Can you work these out from the model? Positions are in its coordinate system, mm. A direction names the side the tool comes from. Give positions to 0.01 mm unless a question says otherwise; leave off trailing zeros. Order: outer loops, then holes, each group sorted by start corner. A loop starts at its lowest first (then second) coordinate and runs counter-clockwise, first axis right, second up. Notation, with made-up numbers: M -12,9 L 32,9 A16 cw 32,36 Z; hole C 11,-28 d1. An arc over 180 degrees is marked long. Use one line per item in the form item = value. Start each with the question number.
1. I want a section at B-B, the plane y = 149. List the corners of the cut face in (x, z) for me (3 decimals).
2. We'd pull the mould along Y, two halves only. Please class faces 6 (the face through (134, 184, 69.85)), 7 (the face through (134, 5.588, 60)), 8 (the face through (134, 12.668, -67)): +Y half, -Y half, draft (parallel to the pull), parting line (faces both ways), or undercut.
3. I want a section at C-C, the plane x = 134.2. Count the separate pieces of the cut face and the enclosed holes in it, and give its area (3 significant figures).
4. I need wall thicknesses on L1, parallel to Y at x = 134, z = 50.8; L2, parallel to Y at x = 134.1, z = 8; L3, parallel to Y at x = 135.45, z = -28.5. Which ranges of each line are inside material? Lowest first, please.
5. I want a section at A-A, the plane y = 34.5. List the corners of the cut face in (x, z) for me (3 decimals), and give its area (3 significant figures).
6. Will these pins go through, and if not, where does the flat tip stop? P1, Ø3, axis at x = 134.5, y = 273.5, coming from the +Z side; P2, Ø1.7, axis at x = 133.5, y = 173, coming from the -Z side; P3, Ø3, axis at x = 133, z = -67, coming from the +Y side.
7. For faces 1 (the face through (134, 24, -30.988)), 2 (the face through (134, 196, 63.5)), 3 (the face through (134, 3, -57.15)), 4 (the face through (134, 108, -69.85)), 5 (the face through (134, 126.682, -67)), which set-ups out of +Z, -Z, +X, -X, +Y, -Y let a thin tool reach every point of the face, with its end or its side?
```python
from build123d import *

# Parameters (mm, degrees)
SKETCH1_W              = 273.05
SKETCH1_H              = 139.7
BOSS_EXTRUDE1_DEPTH    = 5.588
SKETCH2_W              = 273.05
SKETCH2_H              = 139.7
SKETCH2_W_2            = 261.874
SKETCH2_H_2            = 128.524
BOSS_EXTRUDE2_DEPTH    = 298.45
SKETCH3_W              = 6.35
SKETCH3_H              = 16.933333333
SKETCH3_H_2            = 16.933333334
DOOR_SLOT_DEPTH        = 12.7
DOOR_GUIDE_HOLES_REACH = 361.255
SKETCH4_W              = 6.35
SKETCH4_H              = 15.875
LEVER_HOLES_W          = 9.652
LEVER_HOLES_H          = 6.35
LEVER_HOLES_W_2        = 6.35
CUT_EXTRUDE1_DEPTH     = 362.378293578
CUT_EXTRUDE3_REACH     = 416.577
SKETCH8_R              = 3.175
SKETCH16_W             = 327.238778096
SKETCH16_H             = 314.471565403
CUT_EXTRUDE10_DEPTH    = 362.378293578
LEFT_RIGHT_W           = 6.35
LEFT_RIGHT_H           = 5.588
LEFT_RIGHT_W_2         = 12.7
LEFT_RIGHT_H_2         = 12.66825
CUT_EXTRUDE11_DEPTH    = 415.577411883
SKETCH17_R             = 1.5
SKETCH17_W             = 23
SKETCH17_H             = 17.61800007
CUT_EXTRUDE12_DEPTH    = 313.00857951
SKETCH18_W             = 5.588
SKETCH18_H             = 12.192
CUT_EXTRUDE13_DEPTH    = 313.00857951


with BuildPart() as part:
    # Sketch1 → Boss-Extrude1 (new body)
    with BuildSketch(Plane(origin=(0, 0, 0), x_dir=(1, 0, 0), z_dir=(0, 1, 0))):
        Rectangle(SKETCH1_W, SKETCH1_H)
    extrude(amount=BOSS_EXTRUDE1_DEPTH)

    # Sketch2 → Boss-Extrude2 (add)
    with BuildSketch(Plane(origin=(0, 5.588, 0), x_dir=(1, 0, 0), z_dir=(0, 1, 0))):
        Rectangle(SKETCH2_W, SKETCH2_H)
        Rectangle(SKETCH2_W_2, SKETCH2_H_2, mode=Mode.SUBTRACT)
    extrude(amount=BOSS_EXTRUDE2_DEPTH)

    # Sketch3 → Door Slot (cut)
    with BuildSketch(Plane.XY.offset(69.85)):
        with BuildLine():
            Line((-29.337, 282.448), (-29.337, 5.588))
            Line((-29.337, 5.588), (-22.733, 5.588))
            Line((-22.733, 5.588), (-22.733, 291.592))
            Line((-22.733, 291.592), (-42.291, 291.592))
            Line((-42.291, 291.592), (-42.291, 284.988))
            Line((-42.291, 284.988), (-31.877, 284.988))
            ThreePointArc((-31.877, 284.988), (-30.080948776, 284.244051224), (-29.337, 282.448))
        make_face()
        with Locations((-13.208, 80.433333334)):
            Rectangle(SKETCH3_W, SKETCH3_H)
        with Locations((-13.208, 50.8)):
            Rectangle(SKETCH3_W, SKETCH3_H_2)
        with Locations((-13.208, 21.166666667)):
            Rectangle(SKETCH3_W, SKETCH3_H)
    extrude(amount=-DOOR_SLOT_DEPTH, mode=Mode.SUBTRACT)

    # Sketch4 → Door Guide Holes (cut, up to next)
    with BuildSketch(Plane.XY.offset(-64.262), mode=Mode.PRIVATE) as door_guide_holes_sk1:
        with Locations((-45.466, 283.4005)):
            Rectangle(SKETCH4_W, SKETCH4_H)
    door_guide_holes_tool1 = extrude(door_guide_holes_sk1.sketch, amount=-DOOR_GUIDE_HOLES_REACH, mode=Mode.PRIVATE) & part.part
    # Sketch4 → Door Guide Holes (cut, up to next)
    with BuildSketch(Plane.XY.offset(-64.262), mode=Mode.PRIVATE) as door_guide_holes_sk2:
        with Locations((-45.466, 254.8255)):
            Rectangle(SKETCH4_W, SKETCH4_H)
    door_guide_holes_tool2 = extrude(door_guide_holes_sk2.sketch, amount=-DOOR_GUIDE_HOLES_REACH, mode=Mode.PRIVATE) & part.part
    # Sketch4 → Door Guide Holes (cut, up to next)
    with BuildSketch(Plane.XY.offset(-64.262), mode=Mode.PRIVATE) as door_guide_holes_sk3:
        with Locations((-45.466, 226.2505)):
            Rectangle(SKETCH4_W, SKETCH4_H)
    door_guide_holes_tool3 = extrude(door_guide_holes_sk3.sketch, amount=-DOOR_GUIDE_HOLES_REACH, mode=Mode.PRIVATE) & part.part
    # Sketch4 → Door Guide Holes (cut, up to next)
    with BuildSketch(Plane.XY.offset(-64.262), mode=Mode.PRIVATE) as door_guide_holes_sk4:
        with Locations((-45.466, 197.6755)):
            Rectangle(SKETCH4_W, SKETCH4_H)
    door_guide_holes_tool4 = extrude(door_guide_holes_sk4.sketch, amount=-DOOR_GUIDE_HOLES_REACH, mode=Mode.PRIVATE) & part.part
    # Sketch4 → Door Guide Holes (cut, up to next)
    with BuildSketch(Plane.XY.offset(-64.262), mode=Mode.PRIVATE) as door_guide_holes_sk5:
        with Locations((-45.466, 169.1005)):
            Rectangle(SKETCH4_W, SKETCH4_H)
    door_guide_holes_tool5 = extrude(door_guide_holes_sk5.sketch, amount=-DOOR_GUIDE_HOLES_REACH, mode=Mode.PRIVATE) & part.part
    # Sketch4 → Door Guide Holes (cut, up to next)
    with BuildSketch(Plane.XY.offset(-64.262), mode=Mode.PRIVATE) as door_guide_holes_sk6:
        with Locations((-45.466, 140.5255)):
            Rectangle(SKETCH4_W, SKETCH4_H)
    door_guide_holes_tool6 = extrude(door_guide_holes_sk6.sketch, amount=-DOOR_GUIDE_HOLES_REACH, mode=Mode.PRIVATE) & part.part
    # Sketch4 → Door Guide Holes (cut, up to next)
    with BuildSketch(Plane.XY.offset(-64.262), mode=Mode.PRIVATE) as door_guide_holes_sk7:
        with Locations((-45.466, 111.9505)):
            Rectangle(SKETCH4_W, SKETCH4_H)
    door_guide_holes_tool7 = extrude(door_guide_holes_sk7.sketch, amount=-DOOR_GUIDE_HOLES_REACH, mode=Mode.PRIVATE) & part.part
    # Sketch4 → Door Guide Holes (cut, up to next)
    with BuildSketch(Plane.XY.offset(-64.262), mode=Mode.PRIVATE) as door_guide_holes_sk8:
        with Locations((-45.466, 83.3755)):
            Rectangle(SKETCH4_W, SKETCH4_H)
    door_guide_holes_tool8 = extrude(door_guide_holes_sk8.sketch, amount=-DOOR_GUIDE_HOLES_REACH, mode=Mode.PRIVATE) & part.part
    # Sketch4 → Door Guide Holes (cut, up to next)
    with BuildSketch(Plane.XY.offset(-64.262), mode=Mode.PRIVATE) as door_guide_holes_sk9:
        with Locations((-45.466, 54.8005)):
            Rectangle(SKETCH4_W, SKETCH4_H)
    door_guide_holes_tool9 = extrude(door_guide_holes_sk9.sketch, amount=-DOOR_GUIDE_HOLES_REACH, mode=Mode.PRIVATE) & part.part
    # Sketch4 → Door Guide Holes (cut, up to next)
    with BuildSketch(Plane.XY.offset(-64.262), mode=Mode.PRIVATE) as door_guide_holes_sk10:
        with Locations((-45.466, 26.2255)):
            Rectangle(SKETCH4_W, SKETCH4_H)
    door_guide_holes_tool10 = extrude(door_guide_holes_sk10.sketch, amount=-DOOR_GUIDE_HOLES_REACH, mode=Mode.PRIVATE) & part.part
    door_guide_holes_1 = door_guide_holes_tool1.solids().sort_by_distance((-45.466, 283.4005, -64.262))[0]
    add(door_guide_holes_1, mode=Mode.SUBTRACT)
    door_guide_holes_2 = door_guide_holes_tool2.solids().sort_by_distance((-45.466, 254.8255, -64.262))[0]
    add(door_guide_holes_2, mode=Mode.SUBTRACT)
    door_guide_holes_3 = door_guide_holes_tool3.solids().sort_by_distance((-45.466, 226.2505, -64.262))[0]
    add(door_guide_holes_3, mode=Mode.SUBTRACT)
    door_guide_holes_4 = door_guide_holes_tool4.solids().sort_by_distance((-45.466, 197.6755, -64.262))[0]
    add(door_guide_holes_4, mode=Mode.SUBTRACT)
    door_guide_holes_5 = door_guide_holes_tool5.solids().sort_by_distance((-45.466, 169.1005, -64.262))[0]
    add(door_guide_holes_5, mode=Mode.SUBTRACT)
    door_guide_holes_6 = door_guide_holes_tool6.solids().sort_by_distance((-45.466, 140.5255, -64.262))[0]
    add(door_guide_holes_6, mode=Mode.SUBTRACT)
    door_guide_holes_7 = door_guide_holes_tool7.solids().sort_by_distance((-45.466, 111.9505, -64.262))[0]
    add(door_guide_holes_7, mode=Mode.SUBTRACT)
    door_guide_holes_8 = door_guide_holes_tool8.solids().sort_by_distance((-45.466, 83.3755, -64.262))[0]
    add(door_guide_holes_8, mode=Mode.SUBTRACT)
    door_guide_holes_9 = door_guide_holes_tool9.solids().sort_by_distance((-45.466, 54.8005, -64.262))[0]
    add(door_guide_holes_9, mode=Mode.SUBTRACT)
    door_guide_holes_10 = door_guide_holes_tool10.solids().sort_by_distance((-45.466, 26.2255, -64.262))[0]
    add(door_guide_holes_10, mode=Mode.SUBTRACT)
    door_guide_holes = door_guide_holes_1 + door_guide_holes_2 + door_guide_holes_3 + door_guide_holes_4 + door_guide_holes_5 + door_guide_holes_6 + door_guide_holes_7 + door_guide_holes_8 + door_guide_holes_9 + door_guide_holes_10  # Door Guide Holes as one shape, for the pattern or mirror that repeats it

    # Mirror1: Door Guide Holes across plane
    add(door_guide_holes.mirror(Plane.ZY.offset(32.512)), mode=Mode.SUBTRACT)

    # Lever Holes → Cut-Extrude1 (cut, through all)
    with BuildSketch(Plane.XY.offset(69.85)):
        with Locations((54.102, 28.575)):
            Rectangle(LEVER_HOLES_W, LEVER_HOLES_H)
        with Locations((39.3065, 15.875)):
            Rectangle(LEVER_HOLES_W_2, LEVER_HOLES_H)
        with Locations((68.8975, 15.875)):
            Rectangle(LEVER_HOLES_W_2, LEVER_HOLES_H)
    extrude(amount=-CUT_EXTRUDE1_DEPTH, mode=Mode.SUBTRACT)

    # Sketch8 → Cut-Extrude3 (cut, up to next)
    with BuildSketch(Plane.ZY.offset(136.525), mode=Mode.PRIVATE) as cut_extrude3_sk1:
        with Locations((0, 19.05)):
            Circle(SKETCH8_R)
    cut_extrude3_tool1 = extrude(cut_extrude3_sk1.sketch, amount=-CUT_EXTRUDE3_REACH, mode=Mode.PRIVATE) & part.part
    add(cut_extrude3_tool1.solids().sort_by_distance((-136.525, 19.05, 0))[0], mode=Mode.SUBTRACT)

    # Sketch16 → Cut-Extrude10 (cut, through all)
    with BuildSketch(Plane.XY.offset(69.85)):
        with Locations((-32.682389048, 146.802217299)):
            Rectangle(SKETCH16_W, SKETCH16_H)
    extrude(amount=-CUT_EXTRUDE10_DEPTH, mode=Mode.SUBTRACT)

    # Left/Right → Cut-Extrude11 (cut, through all)
    with BuildSketch(Plane.ZY.offset(136.525)):
        with Locations((60.325, 2.794)):
            Rectangle(LEFT_RIGHT_W, LEFT_RIGHT_H)
        with Locations((38.1, 2.794)):
            Rectangle(LEFT_RIGHT_W_2, LEFT_RIGHT_H)
        with Locations((66.675, 19.002375)):
            Rectangle(LEFT_RIGHT_W, LEFT_RIGHT_H_2)
        with Locations((12.7, 2.794)):
            Rectangle(LEFT_RIGHT_W_2, LEFT_RIGHT_H)
        with Locations((66.675, 44.338875)):
            Rectangle(LEFT_RIGHT_W, LEFT_RIGHT_H_2)
        with Locations((-12.7, 2.794)):
            Rectangle(LEFT_RIGHT_W_2, LEFT_RIGHT_H)
        with Locations((66.675, 69.675375)):
            Rectangle(LEFT_RIGHT_W, LEFT_RIGHT_H_2)
        with Locations((-38.1, 2.794)):
            Rectangle(LEFT_RIGHT_W_2, LEFT_RIGHT_H)
        with Locations((66.675, 95.011875)):
            Rectangle(LEFT_RIGHT_W, LEFT_RIGHT_H_2)
        with Locations((-60.325, 2.794)):
            Rectangle(LEFT_RIGHT_W, LEFT_RIGHT_H)
        with Locations((66.675, 120.348375)):
            Rectangle(LEFT_RIGHT_W, LEFT_RIGHT_H_2)
        with Locations((-66.675, 19.002375)):
            Rectangle(LEFT_RIGHT_W, LEFT_RIGHT_H_2)
        with Locations((66.675, 145.684875)):
            Rectangle(LEFT_RIGHT_W, LEFT_RIGHT_H_2)
        with Locations((-66.675, 44.338875)):
            Rectangle(LEFT_RIGHT_W, LEFT_RIGHT_H_2)
        with Locations((66.675, 171.021375)):
            Rectangle(LEFT_RIGHT_W, LEFT_RIGHT_H_2)
        with Locations((-66.675, 69.675375)):
            Rectangle(LEFT_RIGHT_W, LEFT_RIGHT_H_2)
        with Locations((66.675, 196.357875)):
            Rectangle(LEFT_RIGHT_W, LEFT_RIGHT_H_2)
        with Locations((-66.675, 95.011875)):
            Rectangle(LEFT_RIGHT_W, LEFT_RIGHT_H_2)
        with Locations((66.675, 221.694375)):
            Rectangle(LEFT_RIGHT_W, LEFT_RIGHT_H_2)
        with Locations((-66.675, 120.348375)):
            Rectangle(LEFT_RIGHT_W, LEFT_RIGHT_H_2)
        with Locations((66.675, 247.030875)):
            Rectangle(LEFT_RIGHT_W, LEFT_RIGHT_H_2)
        with Locations((-66.675, 145.684875)):
            Rectangle(LEFT_RIGHT_W, LEFT_RIGHT_H_2)
        with Locations((66.675, 272.367375)):
            Rectangle(LEFT_RIGHT_W, LEFT_RIGHT_H_2)
        with Locations((-66.675, 171.021375)):
            Rectangle(LEFT_RIGHT_W, LEFT_RIGHT_H_2)
        with Locations((66.675, 297.703875)):
            Rectangle(LEFT_RIGHT_W, LEFT_RIGHT_H_2)
        with Locations((-66.675, 196.357875)):
            Rectangle(LEFT_RIGHT_W, LEFT_RIGHT_H_2)
        with Locations((-66.675, 221.694375)):
            Rectangle(LEFT_RIGHT_W, LEFT_RIGHT_H_2)
        with Locations((-66.675, 247.030875)):
            Rectangle(LEFT_RIGHT_W, LEFT_RIGHT_H_2)
        with Locations((-66.675, 272.367375)):
            Rectangle(LEFT_RIGHT_W, LEFT_RIGHT_H_2)
        with Locations((-66.675, 297.703875)):
            Rectangle(LEFT_RIGHT_W, LEFT_RIGHT_H_2)
    extrude(amount=-CUT_EXTRUDE11_DEPTH, mode=Mode.SUBTRACT)

    # Sketch17 → Cut-Extrude12 (cut, through all)
    with BuildSketch(Plane(origin=(136.525, 0, 0), x_dir=(0, 0, -1), z_dir=(1, 0, 0))):
        with Locations((-8, 62.088)):
            Circle(SKETCH17_R)
        with Locations((8, 62.088)):
            Circle(SKETCH17_R)
        with Locations((-50.8, 159.894)):
            Circle(SKETCH17_R)
        with Locations((-50.8, 144.144)):
            Circle(SKETCH17_R)
        with Locations(Location((50.8, 144.144, 0), (0, 0, 180))):
            Circle(SKETCH17_R)
        with Locations(Location((50.8, 159.894, 0), (0, 0, 180))):
            Circle(SKETCH17_R)
        with Locations((0, 22.779000035)):
            Rectangle(SKETCH17_W, SKETCH17_H)
    extrude(amount=-CUT_EXTRUDE12_DEPTH, mode=Mode.SUBTRACT)

    # Sketch18 → Cut-Extrude13 (cut, through all)
    with BuildSketch(Plane(origin=(136.525, 0, 0), x_dir=(0, 0, -1), z_dir=(1, 0, 0))):
        with Locations((-28.194, 24.384)):
            Rectangle(SKETCH18_W, SKETCH18_H)
        with Locations((28.194, 24.384)):
            Rectangle(SKETCH18_W, SKETCH18_H)
        Polygon((25.4, 30.48), (25.4, 43.18), (-25.4, 43.18), (-25.4, 30.48), (-25.4, 18.288), (-25.4, 5.588), (-6.35, 5.588), (-6.35, 0), (6.35, 0), (6.35, 5.588), (25.4, 5.588), (25.4, 18.288), align=None)
    extrude(amount=-CUT_EXTRUDE13_DEPTH, mode=Mode.SUBTRACT)


solid = part.part
```
Check result:
q1.outline = M 130.937,-63.5 L 136.525,-63.5 L 136.525,63.5 L 130.937,63.5 Z
q2.face_6 = draft
q2.face_7 = -Y half
q2.face_8 = undercut
q3.separate_pieces = 1
q3.enclosed_holes = 6
q3.area = 38,000 mm2
q4.L1 = 0 to 142.64, 145.64 to 158.39, 161.39 to 304.04
q4.L2 = 43.18 to 60.59, 63.59 to 304.04
q4.L3 = 0 to 18.29, 30.48 to 304.04
q5.outline = M 130.937,-69.85 L 136.525,-69.85 L 136.525,-25.4 L 130.937,-25.4 Z; M 130.937,25.4 L 136.525,25.4 L 136.525,69.85 L 130.937,69.85 Z
q5.area = 497 mm2
q6.P1 = 63.5
q6.P2 = -63.5
q6.P3 = 291.37
q7.face_1 = +X, -X
q7.face_2 = +Z, +X, -X
q7.face_3 = +X, -X, -Y
q7.face_4 = -Z, +X, -X, +Y, -Y
q7.face_5 = -Z, +X, -X
